```python
from build123d import *

# Parameters (mm, degrees)
F0_W     = 10
F0_H     = 10
F1_DEPTH = 10
F2_W     = 4
F2_H     = 4
F3_DEPTH = 2
F4_W     = 4
F4_H     = 4
F6_DEPTH = 2
F5_W     = 4
F5_H     = 4
F7_DEPTH = 2


with BuildPart() as f1:
    # F0 (on Top) → F1 (new body)
    with BuildSketch(Plane.XY):
        Rectangle(F0_W, F0_H)
    extrude(amount=F1_DEPTH)

    # F2 (on face) → F3 (cut)
    with BuildSketch(Plane.YZ.offset(5)):
        with Locations((0, 5)):
            Rectangle(F2_W, F2_H)
    extrude(amount=-F3_DEPTH, mode=Mode.SUBTRACT)

    # F4 (on face) → F6 (cut)
    with BuildSketch(Plane.XZ.offset(5)):
        with Locations((0, 5)):
            Rectangle(F4_W, F4_H)
    extrude(amount=-F6_DEPTH, mode=Mode.SUBTRACT)

    # F5 (on face) → F7 (cut)
    with BuildSketch(Plane.XY.offset(10)):
        Rectangle(F5_W, F5_H)
    extrude(amount=-F7_DEPTH, mode=Mode.SUBTRACT)


solid = f1.part
```
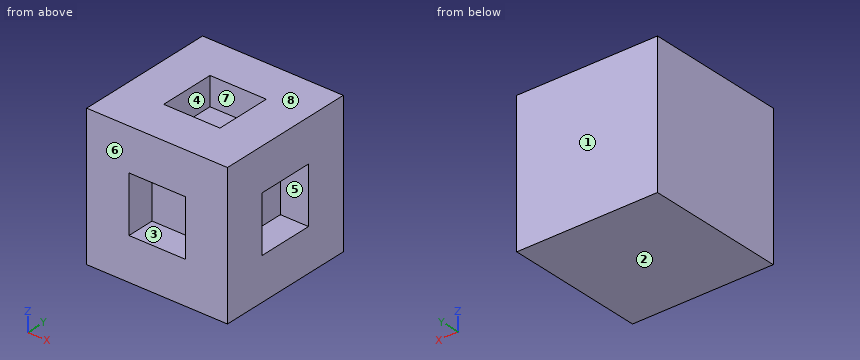
Work out the finished part from the listing and answer in its coordinate system (mm). Face numbers are marked on the shaded views. A direction names the side the tool comes from. Round coordinates to 2 decimals unless told otherwise and drop trailing zeros. Write each loop counter-clockwise with the first axis right and the second up, starting at its lowest first coordinate (ties: lowest second). Pieces come first, ordered by that corner, then holes. Notation, with made-up numbers: (-14, 40.25) -> (36, 40.25) arc R23 cw to (36, 72.25) -> close; hole circle Ø8 at (79.5, 89). An arc over 180 degrees is marked (long way). Write each question's results on one line, items separated by ' | '.
1) The part is cut by section B-B (x = 3.5). Write down the section's boundary in (y, z).
Findings:
outline: (-5, 0) -> (5, 0) -> (5, 10) -> (-5, 10) -> close; hole (-2, 3) -> (2, 3) -> (2, 7) -> (-2, 7) -> close
2) The part is cut by section C-C (x = -1.25). Write down the section's boundary in (y, z).
Findings:
outline: (-5, 0) -> (5, 0) -> (5, 10) -> (2, 10) -> (2, 8) -> (-2, 8) -> (-2, 10) -> (-5, 10) -> (-5, 7) -> (-3, 7) -> (-3, 3) -> (-5, 3) -> close
3) For a pull along Y with two mould halves and no side action, classify the marked faces 6, 7 and 8 as +Y half, -Y half, draft (parallel to the pull), parting line (faces both ways), or undercut.
Findings:
face 6: -Y half | face 7: undercut | face 8: draft
4) Consider line 1 along X through (y, z) = (-3.75, 6.25); line 2 along Y through (x, z) = (-0.25, 5.5). Determine where each line is inside the solid, lowest interval first. Write a range as [from, to].
Findings:
line 1: x = [-5, -2], [2, 5] | line 2: y = [-3, 5]
5) Flat-ended cylindrical pins translate along their axes: pin 1 (3 mm diameter, centred on x = -1, y = 0, fed in from -Z); pin 2 (1.2 mm diameter, centred on x = 0, y = -0.5, fed in from +Z). Find the tip coordinate at first contact, or state that the pin passes through.
Findings:
pin 1: stops at z = 0 | pin 2: stops at z = 8
6) Which of the six approach directions +Z, -Z, +X, -X, +Y, -Y give full straight-line access (tool end or side, diameter ignored) to the marked faces 1, 2, 3, 4 and 5?
Findings:
face 1: +Z, -Z, +X, -X, +Y | face 2: -Z, +X, -X, +Y, -Y | face 3: -Y | face 4: +Z | face 5: +X
7) The part is cut by section A-A (y = -1.5). Write down the section's boundary in (x, z).
Findings:
outline: (-5, 0) -> (5, 0) -> (5, 3) -> (3, 3) -> (3, 7) -> (5, 7) -> (5, 10) -> (2, 10) -> (2, 8) -> (-2, 8) -> (-2, 10) -> (-5, 10) -> close
